```python
from build123d import *

# Parameters (mm, degrees)
SKETCH1_W           = 14.36
SKETCH1_H           = 18.55
BOSS_EXTRUDE1_DEPTH = 1.55
SKETCH2_R           = 1.5
SKETCH2_R_2         = 0.4
CUT_EXTRUDE1_DEPTH  = 2.55
SKETCH5_W           = 2.6
SKETCH5_H           = 1.63
SENSOR_DEPTH        = 0.7
SKETCH6_W           = 1
SKETCH6_H           = 1.5
CAPACITORS1_DEPTH   = 0.3
SKETCH7_W           = 1.22
SKETCH7_H           = 2
CAPACITORS2_DEPTH   = 0.5
SKETCH8_W           = 1.6
SKETCH8_H           = 3
MISC_CHIP1_DEPTH    = 0.6
SKETCH10_W          = 12.6
SKETCH10_H          = 2.5
BOSS_EXTRUDE2_DEPTH = 2.9
SKETCH12_W          = 10.75
SKETCH12_H          = 0.75
BOSS_EXTRUDE3_DEPTH = 5.75


with BuildPart() as part:
    # Sketch1 → Boss-Extrude1 (new body)
    with BuildSketch(Plane(origin=(0, 0, 0), x_dir=(1, 0, 0), z_dir=(0, 1, 0))):
        Rectangle(SKETCH1_W, SKETCH1_H)
    extrude(amount=BOSS_EXTRUDE1_DEPTH)

    # Sketch2 → Cut-Extrude1 (cut, through all)
    with BuildSketch(Plane(origin=(0, 1.55, 0), x_dir=(1, 0, 0), z_dir=(0, 1, 0))):
        with Locations((-4.375, 6.505)):
            Circle(SKETCH2_R)
        with Locations((4.375, 6.505)):
            Circle(SKETCH2_R)
        with Locations((-1.73, -8.275)):
            Circle(SKETCH2_R_2)
        with Locations((1.73, -8.275)):
            Circle(SKETCH2_R_2)
        with Locations((3.46, -8.275)):
            Circle(SKETCH2_R_2)
        with Locations((-3.46, -8.275)):
            Circle(SKETCH2_R_2)
        with Locations((0, -8.275)):
            Circle(SKETCH2_R_2)
    extrude(amount=-CUT_EXTRUDE1_DEPTH, mode=Mode.SUBTRACT)

    # Sketch5 → Sensor (add)
    with BuildSketch(Plane(origin=(0, 1.55, 0), x_dir=(1, 0, 0), z_dir=(0, 1, 0))):
        with Locations((0, 2.36)):
            Rectangle(SKETCH5_W, SKETCH5_H)
    extrude(amount=SENSOR_DEPTH)

    # Sketch6 → Capacitors1 (add)
    with BuildSketch(Plane(origin=(0, 1.55, 0), x_dir=(1, 0, 0), z_dir=(0, 1, 0))):
        with Locations((-5.98, -4.825)):
            Rectangle(SKETCH6_W, SKETCH6_H)
        with Locations((-4.78, -4.825)):
            Rectangle(SKETCH6_W, SKETCH6_H)
        with Locations((-3.58, -4.825)):
            Rectangle(SKETCH6_W, SKETCH6_H)
    extrude(amount=CAPACITORS1_DEPTH)

    # Sketch7 → Capacitors2 (add)
    with BuildSketch(Plane(origin=(0, 1.55, 0), x_dir=(1, 0, 0), z_dir=(0, 1, 0))):
        with Locations((-2.17, -4.825)):
            Rectangle(SKETCH7_W, SKETCH7_H)
        with Locations((-0.65, -4.825)):
            Rectangle(SKETCH7_W, SKETCH7_H)
        with Locations((5.87, -4.825)):
            Rectangle(SKETCH7_W, SKETCH7_H)
    extrude(amount=CAPACITORS2_DEPTH)

    # Sketch8 → misc.chip1 (add)
    with BuildSketch(Plane(origin=(0, 1.55, 0), x_dir=(1, 0, 0), z_dir=(0, 1, 0))):
        with Locations((2.16, -4.825)):
            Rectangle(SKETCH8_W, SKETCH8_H)
    extrude(amount=MISC_CHIP1_DEPTH)

    # Sketch10 → Boss-Extrude2 (add)
    with BuildSketch(Plane.XZ):
        with Locations((0, 8.025)):
            Rectangle(SKETCH10_W, SKETCH10_H)
    extrude(amount=BOSS_EXTRUDE2_DEPTH)

    # Sketch12 → Boss-Extrude3 (add)
    with BuildSketch(Plane.XZ.offset(2.9)):
        with Locations((0, 8.025)):
            Rectangle(SKETCH12_W, SKETCH12_H)
    extrude(amount=BOSS_EXTRUDE3_DEPTH)


solid = part.part
```
Here's how the part is built. I have some questions about the finished solid (model axes, mm). A direction names the side the tool comes from. Give positions to 0.01 mm unless a question says otherwise; leave off trailing zeros. Loops run counter-clockwise (first coordinate to the right, second up) from the corner with the lowest first, then second, coordinate; pieces in that order, holes last. Notation, with made-up numbers: M 62,5 L 86,5 A25 cw 86,38 Z; hole C -39.5,43 d9. An arc over 180 degrees is marked long. Put each result on its own line as item: value. Start each with the question number.
(1) I need wall thicknesses on line 1 along Z through (x, y) = (1.73, 0.75) (3 decimals); line 2 along Z through (x, y) = (0.5, -6); line 3 along Y through (x, z) = (4, 2.25). Which ranges of each line are inside material? Lowest first, please. Write a range as [from, to].
(2) If we mould it in two halves opening along Z, with no side actions, what happens to faces 1 (the flat face through (-1, 2.05, 5)), 2 (the flat face through (0, -6, 8.4)), 3 (the cylindrical face through (-3.547, 0.786, 8.665))? For each: +Z half, -Z half, draft (parallel to the pull), parting line (faces both ways), or undercut.
(3) I want a section at A-A on x = 1.73. Please give me the cut outline in (y, z) (3 decimals), then the cut area to 3 significant figures.
(4) I want a section at D-D on y = -1.5. Please give me the cut outline in (x, z) (3 decimals), then the cut area to 3 significant figures.
(5) Will these pins go through, and if not, where does the flat tip stop? pin 1 Ø1 at (x, y) = (-0.5, -2) entering from -Z (3 decimals); pin 2 Ø0.5 at (x, z) = (2, 4) entering from +Y; pin 3 Ø0.6 at (x, z) = (-2, 5) entering from +Y; pin 4 Ø1 at (y, z) = (-5.5, 6) entering from -X.
(6) I want a section at B-B on x = 3.46. Please give me the cut outline in (y, z) (3 decimals), then the cut area to 3 significant figures.
(7) I want a section at C-C on z = 2. Please give me the cut outline in (x, y).
(8) For faces 4 (the flat face through (-5, 1.85, 5)), 5 (the flat face through (7.18, 1, 0)), 6 (the flat face through (0, -1, 6.775)), 7 (the cylindrical face through (0.18, 0.79, 8.63)), 8 (the flat face through (6, 2.05, 5)), which set-ups out of +Z, -Z, +X, -X, +Y, -Y let a thin tool reach every point of the face, with its end or its side?
Answer block:
1. line 1: [-9.275, 7.875], [8.675, 9.275]
1. line 2: [7.65, 8.4]
1. line 3: [0, 1.55]
2. face 1: draft
2. face 2: +Z half
2. face 3: undercut
3. outline: M -8.65,7.65 L -2.9,7.65 L -2.9,6.775 L 0,6.775 L 0,-9.275 L 1.55,-9.275 L 1.55,3.325 L 2.15,3.325 L 2.15,6.325 L 1.55,6.325 L 1.55,7.875 L 0,7.875 L 0,8.675 L 1.55,8.675 L 1.55,9.275 L -2.9,9.275 L -2.9,8.4 L -8.65,8.4 Z
3. area: 40.9 mm^2
4. outline: M -6.3,6.775 L 6.3,6.775 L 6.3,9.275 L -6.3,9.275 Z
4. area: 31.5 mm^2
5. pin 1: z = 6.775
5. pin 2: y = 2.15
5. pin 3: y = 2.05
5. pin 4: through
6. outline: M -8.65,7.65 L -2.9,7.65 L -2.9,6.775 L 0,6.775 L 0,-5.316 L 1.55,-5.316 L 1.55,7.875 L 0,7.875 L 0,8.675 L 1.55,8.675 L 1.55,9.275 L -2.9,9.275 L -2.9,8.4 L -8.65,8.4 Z; M 0,-9.275 L 1.55,-9.275 L 1.55,-7.694 L 0,-7.694 Z
6. area: 35.4 mm^2
7. outline: M -7.18,0 L 7.18,0 L 7.18,1.55 L -7.18,1.55 Z
8. face 4: +Z, -Z, -X, +Y
8. face 5: +Z, -Z, +X, +Y, -Y
8. face 6: -Z, +X, -X, -Y
8. face 7: +Y
8. face 8: +Z, -Z, +X, +Y
